Check sheet for the modelled part. Datum: model origin and axes. Units: mm. Face numbers are marked on the shaded views. A direction names the side the tool comes from. Coordinates: 2 decimals unless noted, no trailing zeros. Write each loop counter-clockwise with the first axis right and the second up, starting at its lowest first coordinate (ties: lowest second). Pieces come first, ordered by that corner, then holes. Notation, with made-up numbers: (-6, 65) -> (13, 65) arc R16 cw to (13, 87) -> close; hole circle Ø11 at (79, 28.5). An arc over 180 degrees is marked (long way). Put each result on its own line as item: value.
```python
from build123d import *

# Parameters (mm, degrees)
EXTRUDE1_DEPTH  = 57
SKETCH2_R       = 2.75
EXTRUDE2_DEPTH  = 8
EXTRUDE3_DEPTH  = 5
EXTRUDE4_DEPTH  = 50
SKETCH5_R       = 4
EXTRUDE5_DEPTH  = 33
SKETCH6_W       = 30
SKETCH6_H       = 10
EXTRUDE6_DEPTH  = 33
SKETCH7_W       = 50
SKETCH7_H       = 10
EXTRUDE7_DEPTH  = 50
SKETCH10_R      = 1.5
EXTRUDE10_DEPTH = 10
SKETCH11_R      = 2.75
EXTRUDE13_DEPTH = 1
SKETCH12_R      = 15
EXTRUDE14_DEPTH = 10
FILLET2_R       = 5
FILLET3_R       = 5
FILLET4_R       = 10
EXTRUDE15_REACH = 96.553
SKETCH14_W      = 20
SKETCH14_H      = 10
EXTRUDE16_DEPTH = 60
EXTRUDE18_DEPTH = 60
FILLET5_R       = 10
FILLET6_R       = 12
FILLET7_R       = 3
FILLET8_R       = 3
FILLET9_R       = 3


# Some blends are built 0.0001 mm under size
with BuildPart() as part:
    # Sketch1 → Extrude1 (new body)
    with BuildSketch(Plane.XY):
        with BuildLine():
            Line((73.499997202, -17), (73.499997202, 0))
            Line((73.499997202, 0), (39, 0))
            Line((39, 0), (39, -17))
            Line((39, -17), (43.389340395, -17))
            ThreePointArc((43.389340395, -17), (48.49587093, -14.994566191), (53.602401465, -17))
            Line((53.602401465, -17), (73.499997202, -17))
        make_face()
    extrude(amount=-EXTRUDE1_DEPTH)

    # Sketch2 → Extrude2 (add)
    with BuildSketch(Plane.XY):
        with BuildLine():
            Line((57.95839, -23.293955), (57.95839, -17))
            Line((57.95839, -17), (71.309471167, -17))
            ThreePointArc((71.309471167, -17), (69.395977388, -29.48722516), (57.767354943, -24.550891432))
            ThreePointArc((57.767354943, -24.550891432), (57.883931975, -23.925623937), (57.95839, -23.293955))
        make_face()
        with Locations((65.5, -22.5)):
            Circle(SKETCH2_R, mode=Mode.SUBTRACT)
    extrude(amount=-EXTRUDE2_DEPTH)

    # Sketch3 → Extrude3 (cut)
    with BuildSketch(Plane(origin=(0, 0, -8), x_dir=(-1, 0, 0), z_dir=(0, 0, -1))):
        Polygon((-69.5, -20.190598923), (-65.5, -17.881197846), (-61.5, -20.190598923), (-61.5, -24.809401077), (-65.5, -27.118802154), (-69.5, -24.809401077), align=None)
    extrude(amount=-EXTRUDE3_DEPTH, mode=Mode.SUBTRACT)

    # Sketch4 → Extrude4 (add)
    with BuildSketch(Plane.XY):
        with BuildLine():
            Line((39, -17), (39, -22.5))
            ThreePointArc((39, -22.5), (45.271742795, -31.43055539), (55.801591252, -28.564919557))
            Line((55.801591252, -28.564919557), (54.269524764, -27.292339419))
            ThreePointArc((54.269524764, -27.292339419), (43.338902241, -27.950290613), (43.389340395, -17))
            Line((43.389340395, -17), (39, -17))
        make_face()
        with BuildLine():
            Line((56.876362299, -26.964085637), (55.118731957, -26.027376827))
            ThreePointArc((55.118731957, -26.027376827), (55.896414133, -21.25571178), (53.602401465, -17))
            Line((53.602401465, -17), (57.95839, -17))
            Line((57.95839, -17), (57.95839, -23.293955))
            ThreePointArc((57.95839, -23.293955), (57.60414849, -25.184084529), (56.876362299, -26.964085637))
        make_face()
    extrude(amount=-EXTRUDE4_DEPTH)

    # Sketch5 → Extrude5 (cut)
    with BuildSketch(Plane(origin=(73.499997202, 0, 0), x_dir=(0, 0, -1), z_dir=(1, 0, 0))):
        with Locations((6, -8.5)):
            Circle(SKETCH5_R)
        with Locations((51, -8.5)):
            Circle(SKETCH5_R)
    extrude(amount=-EXTRUDE5_DEPTH, mode=Mode.SUBTRACT)

    # Sketch6 → Extrude6 (cut)
    with BuildSketch(Plane(origin=(73.499997202, 0, 0), x_dir=(0, 0, -1), z_dir=(1, 0, 0))):
        with Locations((28.5, -8.5)):
            Rectangle(SKETCH6_W, SKETCH6_H)
    extrude(amount=-EXTRUDE6_DEPTH, mode=Mode.SUBTRACT)

    # Sketch7 → Extrude7 (add)
    with BuildSketch(Plane.ZY.offset(-39)):
        with Locations((-25, -5)):
            Rectangle(SKETCH7_W, SKETCH7_H)
    extrude(amount=EXTRUDE7_DEPTH)

    # Sketch10 → Extrude10 (cut)
    with BuildSketch(Plane.XZ.offset(10)):
        with Locations((-4.599204374, -45)):
            Circle(SKETCH10_R)
        with Locations((26.400795626, -45)):
            Circle(SKETCH10_R)
        with Locations((26.400795626, -14)):
            Circle(SKETCH10_R)
        with Locations((-4.599204374, -14)):
            Circle(SKETCH10_R)
    extrude(amount=-EXTRUDE10_DEPTH, mode=Mode.SUBTRACT)

    # Sketch11 → Extrude13 (cut)
    with BuildSketch(Plane.XZ.offset(10)):
        with Locations((-4.599204374, -14)):
            Circle(SKETCH11_R)
        with Locations((26.400795626, -14)):
            Circle(SKETCH11_R)
        with Locations((26.400795626, -45)):
            Circle(SKETCH11_R)
    extrude(amount=-EXTRUDE13_DEPTH, mode=Mode.SUBTRACT)

    # Sketch12 → Extrude14 (cut)
    with BuildSketch(Plane.XZ.offset(10)):
        with Locations((10.900795626, -30.5)):
            Circle(SKETCH12_R)
    extrude(amount=-EXTRUDE14_DEPTH, mode=Mode.SUBTRACT)

    # Fillet2
    fillet2_edges = [part.edges().sort_by_distance(p)[0] for p in [
        (48.49587093, -14.994566191, -57),
        (63.551199334, -17, -57),
        (41.194670197, -17, -57),
    ]]
    fillet(fillet2_edges, radius=FILLET2_R)

    # Fillet3
    fillet3_edges = [part.edges().sort_by_distance(p)[0] for p in [
        (56.249998601, 0, -57),
    ]]
    fillet(fillet3_edges, radius=FILLET3_R)

    # Fillet4
    fillet4_edges = [part.edges().sort_by_distance(p)[0] for p in [
        (56.999997202, -13.5, -43.5),
    ]]
    fillet(fillet4_edges, radius=FILLET4_R - 0.0001)  # a hair under: the kernel refuses the full size

    # Extrude15: up to this face of the body (flat: up to its plane)
    extrude15_end = Plane(part.part.faces().sort_by_distance((35.938109504, 0, -24.375937497))[0])
    # Sketch13 → Extrude15 (cut, up to the picked face)
    with BuildSketch(Plane.XZ.offset(17), mode=Mode.PRIVATE) as extrude15_sk1:
        with BuildLine():
            Line((57.95839, -16.137451745), (57.95839, -43.862548255))
            ThreePointArc((57.95839, -43.862548255), (69.999997202, -30), (57.95839, -16.137451745))
        make_face()
    extrude15_tool1 = split(extrude(extrude15_sk1.sketch, amount=-EXTRUDE15_REACH, mode=Mode.PRIVATE), bisect_by=extrude15_end, keep=Keep.BOTH, mode=Mode.PRIVATE)
    add(extrude15_tool1.solids().sort_by(Axis((63.013259, -17, -30), (0, 1, 0)))[0], mode=Mode.SUBTRACT)

    # Sketch14 → Extrude16 (cut)
    with BuildSketch(Plane(origin=(40.499997202, 0, 0), x_dir=(0, 0, -1), z_dir=(1, 0, 0))):
        with Locations((30, -8.5)):
            Rectangle(SKETCH14_W, SKETCH14_H)
    extrude(amount=-EXTRUDE16_DEPTH, mode=Mode.SUBTRACT)

    # Sketch15 → Extrude18 (cut)
    with BuildSketch(Plane(origin=(0, 0, 0), x_dir=(1, 0, 0), z_dir=(0, 1, 0))):
        Polygon((2.11392048, 20), (-12.43887347, 20), (-12.43887347, 50), (20.496397049, 50), (20.496397049, 40), (2.11392048, 40), align=None)
    extrude(amount=-EXTRUDE18_DEPTH, mode=Mode.SUBTRACT)

    # Fillet5
    # the kernel refuses this fillet: 10 mm, written as the material it adds along each edge
    with BuildSketch(Plane(origin=(73.499997202, -13.5, -13.5), x_dir=(0, 1, 0), z_dir=(-1, 0, 0))) as fillet5_piece_1_section:
        with BuildLine():
            CenterArc((FILLET5_R, FILLET5_R), FILLET5_R, 180, 90)
            Line((0, FILLET5_R), (0, 0))
            Line((0, 0), (FILLET5_R, 0))
        make_face()
    fillet5_piece_1 = extrude(amount=33, mode=Mode.PRIVATE)
    fillet5_piece_1 = split(fillet5_piece_1, bisect_by=Plane(origin=(57.95839, -11.020059701, -15.351239597), z_dir=(1, 0, 0)), keep=Keep.TOP, mode=Mode.PRIVATE)
    fillet5_piece_1 = fillet5_piece_1 - Plane(origin=(55.999766898, -11.020059701, -30), x_dir=(0.13989934874108464, 0, -0.9901657296744927), z_dir=(0, -1, 0)) * Cylinder(14.000230304, 106, mode=Mode.PRIVATE)
    add(fillet5_piece_1)
    with BuildSketch(Plane(origin=(73.499997202, -13.5, -13.5), x_dir=(0, 1, 0), z_dir=(-1, 0, 0))) as fillet5_piece_2_section:
        with BuildLine():
            CenterArc((FILLET5_R, FILLET5_R), FILLET5_R, 180, 90)
            Line((0, FILLET5_R), (0, 0))
            Line((0, 0), (FILLET5_R, 0))
        make_face()
    fillet5_piece_2 = extrude(amount=33, mode=Mode.PRIVATE)
    fillet5_piece_2 = split(fillet5_piece_2, bisect_by=Plane(origin=(57.95839, -10.883667804, -15.13209824), z_dir=(-1, 0, 0)), keep=Keep.TOP, mode=Mode.PRIVATE)
    fillet5_piece_2 = fillet5_piece_2 - Plane(origin=(55.999766898, -10.883667804, -30), x_dir=(0.13989934874108464, 0, -0.9901657296744927), z_dir=(0, -1, 0)) * Cylinder(14.000230304, 106, mode=Mode.PRIVATE)
    add(fillet5_piece_2)
    with BuildSketch(Plane(origin=(73.499997202, -13.5, -13.5), x_dir=(0, 1, 0), z_dir=(-1, 0, 0))) as fillet5_piece_3_section:
        with BuildLine():
            CenterArc((FILLET5_R, FILLET5_R), FILLET5_R, 180, 90)
            Line((0, FILLET5_R), (0, 0))
            Line((0, 0), (FILLET5_R, 0))
        make_face()
    fillet5_piece_3 = extrude(amount=33, mode=Mode.PRIVATE)
    fillet5_piece_3 = split(fillet5_piece_3, bisect_by=Plane(origin=(57.95839, -12.859707332, -18.675298705), z_dir=(-1, 0, 0)), keep=Keep.TOP, mode=Mode.PRIVATE)
    fillet5_piece_3 = fillet5_piece_3 & Plane(origin=(55.999766898, -12.859707332, -30), x_dir=(0.13989934874108464, 0, -0.9901657296744927), z_dir=(0, -1, 0)) * Cylinder(14.000230304, 106, mode=Mode.PRIVATE)
    add(fillet5_piece_3)
    with BuildSketch(Plane(origin=(73.499997202, -13.5, -13.5), x_dir=(0, 1, 0), z_dir=(-1, 0, 0))) as fillet5_piece_4_section:
        with BuildLine():
            CenterArc((FILLET5_R, FILLET5_R), FILLET5_R, 180, 90)
            Line((0, FILLET5_R), (0, 0))
            Line((0, 0), (FILLET5_R, 0))
        make_face()
    fillet5_piece_4 = extrude(amount=58, mode=Mode.PRIVATE)
    fillet5_piece_4 = split(fillet5_piece_4, bisect_by=Plane(origin=(40.499997202, -11.236048857, -15.763951143), z_dir=(-1, 0, 0)), keep=Keep.TOP, mode=Mode.PRIVATE)
    fillet5_piece_4 = split(fillet5_piece_4, bisect_by=Plane(origin=(39, -11.236048857, -15.763951143), z_dir=(1, 0, 0)), keep=Keep.TOP, mode=Mode.PRIVATE)
    add(fillet5_piece_4)

    # Fillet6
    fillet6_edges = [part.edges().sort_by_distance(p)[0] for p in [
        (0.188652983, -5, -20),
        (20.496397049, -5, -42.029285899),
    ]]
    fillet(fillet6_edges, radius=FILLET6_R)

    # Fillet7
    # the kernel refuses this fillet: 3 mm, written as the material it takes off along each edge
    with BuildSketch(Plane(origin=(40.499997202, -18.59939602, -40), x_dir=(-1, 0, 0), z_dir=(0, 1, 0))) as fillet7_piece_1_section:
        with BuildLine():
            CenterArc((FILLET7_R, -FILLET7_R), FILLET7_R, 90, 90)
            Line((0, -FILLET7_R), (0, 0))
            Line((0, 0), (FILLET7_R, 0))
        make_face()
    fillet7_piece_1 = extrude(amount=15.09939602, mode=Mode.PRIVATE)
    fillet7_piece_1 = split(fillet7_piece_1, bisect_by=Plane(origin=(39.991722384, -13.5, -40.797398057), z_dir=(0, 1, 0)), keep=Keep.TOP, mode=Mode.PRIVATE)
    add(fillet7_piece_1, mode=Mode.SUBTRACT)
    with BuildSketch(Plane(origin=(40.499997202, -3.5, -20), x_dir=(-1, 0, 0), z_dir=(0, -1, 0))) as fillet7_piece_2_section:
        with BuildLine():
            CenterArc((FILLET7_R, -FILLET7_R), FILLET7_R, 90, 90)
            Line((0, -FILLET7_R), (0, 0))
            Line((0, 0), (FILLET7_R, 0))
        make_face()
    fillet7_piece_2 = extrude(amount=16.867496998, mode=Mode.PRIVATE)
    fillet7_piece_2 = fillet7_piece_2 & Plane(origin=(38.630208494, -3.5, -23.5), x_dir=(0, 1, 0), z_dir=(1, 0, 0)) * Cylinder(10, 46, mode=Mode.PRIVATE)
    add(fillet7_piece_2, mode=Mode.SUBTRACT)

    # Fillet8
    fillet8_edges = [part.edges().sort_by_distance(p)[0] for p in [
        (-11, -5, -20),
    ]]
    fillet(fillet8_edges, radius=FILLET8_R)

    # Fillet9
    fillet9_edges = [part.edges().sort_by_distance(p)[0] for p in [
        (20.496397049, -5, -50),
    ]]
    fillet(fillet9_edges, radius=FILLET9_R)


solid = part.part
```
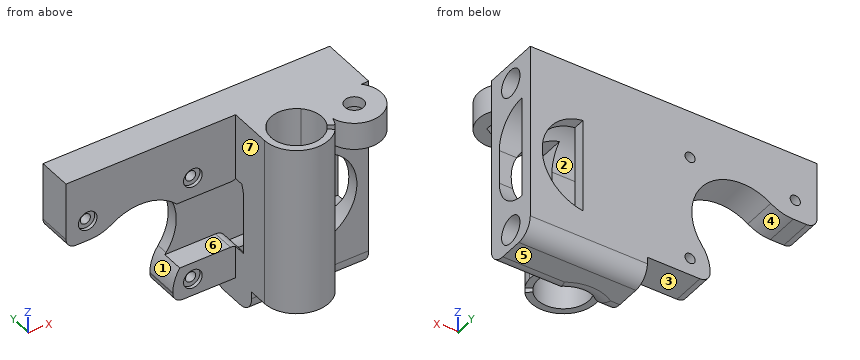
Q1. Cross-section at B-B (y = -21.5). Record the cut outline in (x, z), plus the area to 3 significant figures.
Recorded:
outline: (39, -50) -> (41.06, -50) -> (41.06, 0) -> (39, 0) -> close; (55.93, -50) -> (57.96, -50) -> (57.96, -8) -> (61.5, -8) -> (61.5, -3) -> (62.94, -3) -> (62.94, 0) -> (55.93, 0) -> close; (68.06, -3) -> (69.5, -3) -> (69.5, -8) -> (73.44, -8) -> (73.44, 0) -> (68.06, 0) -> close
area: 273 mm2
Q2. Material ranges on line 1 along X through (y, z) = (-23, -16); line 2 along Y through (x, z) = (70, -24.5); line 3 along Y through (x, z) = (49, -3.5), recorded low to high.
Recorded:
line 1: x = 39.01 to 41.01, 55.98 to 57.96
line 2: y = -17 to -13.5, -3.5 to 0
line 3: y = -31.98 to -29.99, -15.01 to -11.62, -5.38 to 0
Q3. Tool access check on the marked faces 1, 2, 3 and 4. Record the directions out of +Z, -Z, +X, -X, +Y, -Y that give a thin tool (end or side, any length) a straight path to the whole face; none if there is none.
Recorded:
face 1: -X, +Y, -Y
face 2: +X
face 3: -Z, -X, +Y, -Y
face 4: -Z, +Y, -Y
Q4. Cross-section at C-C (z = -51). Record the cut outline in (x, y), plus the area to 3 significant figures.
Recorded:
outline: (39, -17) -> (43.39, -17) arc R7.5 cw to (53.6, -17) -> (73.5, -17) -> (73.5, -12.5) -> (40.5, -12.5) -> (40.5, -4.5) -> (73.5, -4.5) -> (73.5, 0) -> (39, 0) -> close
area: 308 mm2
Q5. Depth check by flat-ended pin: P1, Ø8, axis at y = -24, z = -46.5, coming from the -X side; P2, Ø4, axis at y = -10, z = -5, coming from the +X side; P3, Ø2, axis at x = -5.5, y = -4, coming from the -Z side. Enter the tip coordinate at first touch or a pass-through.
Recorded:
P1: stops at x = 39
P2: stops at x = 40.5
P3: stops at z = -20
Q6. Cross-section at A-A (z = -28). Record the cut outline in (x, y), plus the area to 3 significant figures.
Recorded:
outline: (25.69, -3.5) -> (57.96, -3.5) -> (57.96, 0) -> (25.69, 0) -> close; (39, -22.5) arc R9.5 ccw to (55.8, -28.56) -> (54.27, -27.29) arc R7.5 cw (long way) to (55.12, -26.03) -> (56.88, -26.96) arc R9.5 ccw to (57.96, -23.29) -> (57.96, -13.5) -> (39, -13.5) -> close; (69.86, -17) -> (73.5, -17) -> (73.5, -13.5) -> (69.86, -13.5) -> close; (69.86, -3.5) -> (73.5, -3.5) -> (73.5, 0) -> (69.86, 0) -> close
area: 270 mm2
Q7. Mould release check, pull along Z, two halves, no side actions. Record for the marked faces 5, 6 and 7: released by +Z, released by -Z, zero draft, split by the parting line, or undercut.
Recorded:
face 5: released by -Z
face 6: undercut
face 7: zero draft
Q8. Cross-section at D-D (x = 51). State how many separate pieces and enclosed holes the cut face has, plus the area to 3 significant figures.
Recorded:
separate pieces: 2
enclosed holes: 3
area: 615 mm2
